Can you work these out from the model? Positions are in its coordinate system, mm. Face numbers are marked on the shaded views. A direction names the side the tool comes from. Give positions to 0.01 mm unless a question says otherwise; leave off trailing zeros. Write each loop counter-clockwise with the first axis right and the second up, starting at its lowest first coordinate (ties: lowest second). Pieces come first, ordered by that corner, then holes.
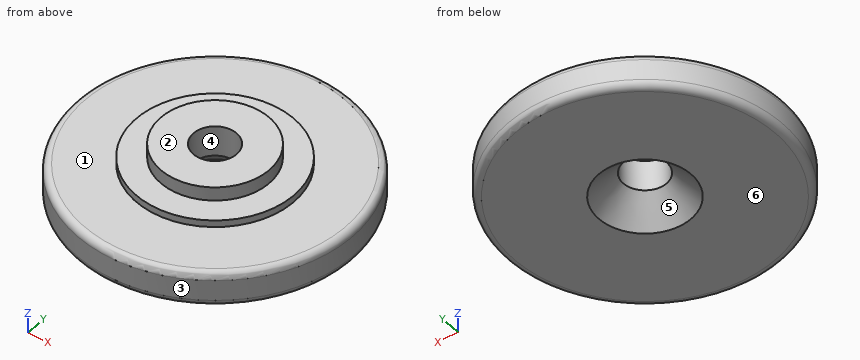
```python
from build123d import *

# Parameters (mm, degrees)
F0_R           = 10
F1_DEPTH       = 2.5
F2_R           = 3.95
F3_DEPTH       = 1.5
F2_R_2         = 5.75
F4_DEPTH       = 0.5
F5_R           = 0.5
F6_D           = 3.15
F6_CSINK_D     = 6.72
F6_CSINK_ANGLE = 90


with BuildPart() as f1:
    # F0 (on Top) → F1 (new body)
    with BuildSketch(Plane.XY):
        Circle(F0_R)
    extrude(amount=F1_DEPTH)

    # F2 (on face) → F3 (join)
    with BuildSketch(Plane.XY.offset(2.5)):
        Circle(F2_R)
    extrude(amount=F3_DEPTH)

    # F2 (on face) → F4 (join)
    with BuildSketch(Plane.XY.offset(2.5)):
        Circle(F2_R_2)
        Circle(F2_R, mode=Mode.SUBTRACT)
    extrude(amount=F4_DEPTH)

    # F5
    f5_edges = [f1.edges().sort_by_distance(p)[0] for p in [
        (-10, 0, 0),
        (-10, 0, 2.5),
    ]]
    fillet(f5_edges, radius=F5_R)

    # F6 (through all)
    with Locations(Plane(origin=(0, 0, 0), x_dir=(1, 0, 0), z_dir=(0, 0, -1))):
        with Locations((0, 0)):
            CounterSinkHole(F6_D / 2, F6_CSINK_D / 2, counter_sink_angle=F6_CSINK_ANGLE)


solid = f1.part
```
1) For pin 1 Ø3 at (x, y) = (7.5, 0.5) entering from +Z; pin 2 Ø4 at (x, y) = (0, 0) entering from -Z; pin 3 Ø4 at (x, y) = (-2.5, -6.5) entering from +Z, each with a flat end and sliding along its axis, tell me the tip position at first contact or that it passes through.
Values follow:
pin 1: stops at z = 2.5
pin 2: stops at z = 1.36
pin 3: stops at z = 3
2) Please list where these lines run through material, in increasing order: L1, parallel to Y at x = 0, z = 2.8 (3 decimals); L2, parallel to Y at x = 0, z = 3.45 (3 decimals); L3, parallel to Z at x = -2.5, y = -4.
Values follow:
L1: y = -5.75 to -1.575, 1.575 to 5.75
L2: y = -3.95 to -1.575, 1.575 to 3.95
L3: z = 0 to 3
3) Suppose I cut it at A-A on y = 0. Write out the boundary of the cut face in (x, z) (3 decimals), plus the area to 3 significant figures.
Values follow:
outline: (-10, 0.5) arc R0.5 ccw to (-9.5, 0) - (-3.36, 0) - (-1.575, 1.785) - (-1.575, 4) - (-3.95, 4) - (-3.95, 3) - (-5.75, 3) - (-5.75, 2.5) - (-9.5, 2.5) arc R0.5 ccw to (-10, 2) - close; (1.575, 1.785) - (3.36, 0) - (9.5, 0) arc R0.5 ccw to (10, 0.5) - (10, 2) arc R0.5 ccw to (9.5, 2.5) - (5.75, 2.5) - (5.75, 3) - (3.95, 3) - (3.95, 4) - (1.575, 4) - close
area: 47.6 mm2
4) Suppose I cut it at C-C on z = 3.5. Write out the boundary of the cut face in (x, y) (3 decimals).
Values follow:
outline: circle Ø7.9 at (0, 0); hole circle Ø3.15 at (0, 0)
5) If we mould it in two halves opening along X, with no side actions, what happens to the marked faces 3, 4, 5 and 6? For each: +X half, -X half, draft (parallel to the pull), parting line (faces both ways), or undercut.
Values follow:
face 3: parting line
face 4: undercut
face 5: undercut
face 6: draft
6) For the marked faces 1 and 2, which set-ups out of +Z, -Z, +X, -X, +Y, -Y let a thin tool reach every point of the face, with its end or its side?
Values follow:
face 1: +Z
face 2: +Z, +X, -X, +Y, -Y
